```python
from build123d import *

# Parameters (mm, degrees)
F0_W     = 36
F0_H     = 36
F1_DEPTH = 500
F3_DEPTH = 40.001


# Not quite as in the source:
# - a pattern or mirror of a feature is missing from the dataset's text; its kind, count and spacing are read off the source's solid


with BuildPart() as f1:
    # F0 (on Top) → F1 (new body, symmetric)
    with BuildSketch(Plane.XY):
        with BuildLine():
            Line((17, 20), (-17, 20))
            ThreePointArc((-17, 20), (-19.1213203436, 19.1213203436), (-20, 17))
            Line((-20, 17), (-20, -17))
            ThreePointArc((-20, -17), (-19.1213203436, -19.1213203436), (-17, -20))
            Line((-17, -20), (17, -20))
            ThreePointArc((17, -20), (19.1213203436, -19.1213203436), (20, -17))
            Line((20, -17), (20, 17))
            ThreePointArc((20, 17), (19.1213203436, 19.1213203436), (17, 20))
        make_face()
        Rectangle(F0_W, F0_H, mode=Mode.SUBTRACT)
    extrude(amount=F1_DEPTH, both=True)

    # F2 (on face) → F3 (cut, through all)
    with BuildSketch(Plane.XZ.offset(20)):
        Polygon((20, 500), (-20, 500), (20, 460), align=None)
    f3 = extrude(amount=-F3_DEPTH, mode=Mode.SUBTRACT)

    # F3_copies: F3 across plane
    add(f3.mirror(Plane(origin=(0, 0, 0), x_dir=(-1, 0, 0), z_dir=(0, 0, -1))), mode=Mode.SUBTRACT)


solid = f1.part
```
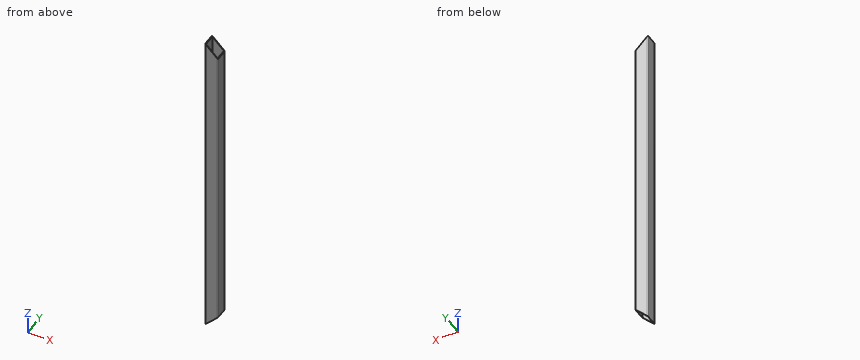
Part model, mm, in its own coordinate system. Round coordinates to 2 decimals unless told otherwise and drop trailing zeros. Loops run counter-clockwise (first coordinate to the right, second up) from the corner with the lowest first, then second, coordinate; pieces in that order, holes last. Notation, with made-up numbers: (-1, 3) -> (56, 3) arc R12 cw to (56, 8) -> close; hole circle Ø7 at (27.25, 34.5). An arc over 180 degrees is marked (long way). Use CSV: the item, a comma, the result in double quotes. Start each with the question number.
1) Cut at A-A, the plane y = 10.5. Write the cut outline in (x, z).
2) Wall check: L1, parallel to X at y = -14, z = -300. Give the ranges that are in metal, low to high. Write a range as [from, to].
3) Cut at B-B, the plane x = -2. Write the cut outline in (y, z).
4) Cut at C-C, the plane z = -220. Write the cut outline in (x, y).
Determined:
1,outline,"(-20, -500) -> (-18, -498) -> (-18, 498) -> (-20, 500) -> close; (18, -462) -> (20, -460) -> (20, 460) -> (18, 462) -> close"
2,L1,"x = [-20, -18], [18, 20]"
3,outline,"(-20, -482) -> (-18, -482) -> (-18, 482) -> (-20, 482) -> close; (18, -482) -> (20, -482) -> (20, 482) -> (18, 482) -> close"
4,outline,"(-20, -17) arc R3 ccw to (-17, -20) -> (17, -20) arc R3 ccw to (20, -17) -> (20, 17) arc R3 ccw to (17, 20) -> (-17, 20) arc R3 ccw to (-20, 17) -> close; hole (-18, -18) -> (18, -18) -> (18, 18) -> (-18, 18) -> close"
